Autodesk Inventor part; units mm, degrees
ref_plane "YZ Plane" through (0, 0, 0) normal (1, 0, 0) x (0, 1, 0)
ref_plane "XZ Plane" through (0, 0, 0) normal (0, 1, 0) x (-1, 0, 0)
ref_plane "XY Plane" through (0, 0, 0) normal (0, 0, 1) x (1, 0, 0)
sketch "Эскиз1" plane through (0, 0, 0) normal (0, 1, 0) x (-1, 0, 0)
  line L0 (0, 0) -> (36.1, 0)
  line L1 (36.1, 0) -> (36.1, -7)
  line L2 (36.1, -7) -> (0, -7)
  line L3 (0, -7) -> (0, 0)
  line L4 (36.1, -7) -> (31.1, -7)
  line L5 (31.1, -7) -> (31.1, -12)
  line L6 (31.1, -12) -> (36.1, -12)
  line L7 (36.1, -12) -> (36.1, -7)
  line L8 (36.1, -12) -> (40.1, -12)
  line L9 (40.1, -12) -> (40.1, -5)
  line L10 (40.1, -5) -> (36.1, -5)
  line L11 (36.1, -5) -> (36.1, -12)
  line L12 (18.05, 0) -> (18.05, -7) construction
  line L13 (0, -7) -> (5, -7)
  line L14 (5, -7) -> (5, -12)
  line L15 (5, -12) -> (0, -12)
  line L16 (0, -12) -> (0, -7)
  line L17 (0, -12) -> (-4, -12)
  line L18 (-4, -12) -> (-4, -5)
  line L19 (-4, -5) -> (0, -5)
  line L20 (0, -5) -> (0, -12)
  point P0 (31.1, -7)
  point P1 (0, -5)
  point P2 (36.1, -5)
  dimension "d0" = 36.1
  dimension "d1" = 7
  dimension "d12" = 5
  dimension "d13" = 5
  dimension "d14" = 4
  dimension "d15" = 7
extrude "Выдавливание1" add sketch "Эскиз1" along normal blind 4
sketch "Эскиз2" plane through (0, 0, 0) normal (0, -1, 0) x (1, 0, 0)
  line L0 (-36.1, 0) -> (0, 0) construction
  line L1 (-18.05, 0) -> (-18.05, -7) construction
  line L2 (-5, -7) -> (-31.1, -7) construction
  line L3 (-32.8, -3.5) -> (-3.3, -3.5) construction
  point P0 (-35.5, 0)
  point P1 (0, -7)
  point P2 (-35.5, -7)
  point P3 (-18.05, -3.5)
  dimension "d4" = 29.5
hole "Отверстие1" at (-32.8, 0, -3.5) at (-3.3, 0, -3.5) direction (0, 1, 0) diameter 3.2 end through all countersink diameter 6 countersink angle 90
sketch "Эскиз3" plane through (0, 4, 0) normal (0, 1, 0) x (1, 0, 0)
  line L0 (-40.1, 5) -> (-36.1, 5)
  line L1 (-36.1, 5) -> (-36.1, 12)
  line L2 (-31.1, 12) -> (-40.1, 12)
  line L3 (0, 5) -> (4, 5)
  line L4 (0, 5) -> (0, 12)
  line L5 (4, 12) -> (-5, 12)
  line L6 (4, 5) -> (4, 12)
  line L7 (-40.1, 12) -> (-40.1, 5)
  point P0 (0, 0)
extrude "Выдавливание2" add sketch "Эскиз3" along normal blind 11.05
fillet "Сопряжение1" radius 3.5 4 edges at (-38.1, 15.05, -5) (-38.1, 15.05, -12) (2, 15.05, -5) (2, 15.05, -12)
sketch "Эскиз5" plane through (-40.1, 0, -12) normal (-1, 0, 0) x (0, 0, 1)
  arc A0 (7, 11.55) -> (0, 11.55) centre (3.5, 11.55) ccw
  arc A1 (7, 11.55) -> (0, 11.55) centre (3.5, 11.55) ccw
  point P0 (12, 0)
hole "Отверстие2" at (-40.1, 11.55, -8.5) direction (1, 0, 0) diameter 3.1 depth 3.5
sketch "Эскиз6" plane through (4, 0, -5) normal (1, 0, 0) x (0, 0, -1)
  arc A0 (7, 11.55) -> (0, 11.55) centre (3.5, 11.55) ccw
  point P0 (-5, 0)
hole "Отверстие3" at (4, 11.55, -8.5) direction (-1, 0, 0) diameter 3.1 depth 3.5
sketch "Эскиз7" plane through (-40.1, 0, -12) normal (-1, 0, 0) x (0, 0, 1)
  circle A0 centre (3.5, 11.55) radius 1.55
  line L0 (0.7, 13.1666) -> (3.5, 14.7832)
  line L1 (3.5, 14.7832) -> (6.3, 13.1666)
  line L2 (6.3, 13.1666) -> (6.3, 9.9334)
  line L3 (6.3, 9.9334) -> (3.5, 8.3168)
  line L4 (3.5, 8.3168) -> (0.7, 9.9334)
  line L5 (0.7, 9.9334) -> (0.7, 13.1666)
  line L6 (0, 0) -> (0, 11.55)
  line L7 (0.7, 9.9334) -> (6.3, 9.9334)
  line L8 (6.3, 9.9334) -> (6.3, 0)
  line L9 (6.3, 0) -> (0.7, 0)
  line L10 (0.7, 0) -> (0.7, 9.9334)
  line L11 (0, 0) -> (7, 0)
  point P0 (12, 0)
  point P1 (3.5, 11.55)
  dimension "d33" = 5.6
extrude "Выдавливание3" cut sketch "Эскиз7" along normal blind 3 from surface at -3.5 contours A0 | L0 L1 L2 L7 L5 | L7 L3 L4 | L4 L3 L8 L9 L10
extrude "Выдавливание4" cut sketch "Эскиз7" against normal blind 3 from surface at -40.6 contours A0 | L0 L1 L2 L7 L5 | L7 L3 L4 | L4 L3 L8 L9 L10
sketch "Эскиз8" plane through (0, 4, 0) normal (0, 1, 0) x (1, 0, 0)
  line L0 (-31.1, 7) -> (-31.1, 12)
  line L1 (-31.1, 12) -> (-36.1, 12)
  line L2 (-36.1, 12) -> (-36.1, 10.5)
  line L3 (-36.1, 10.5) -> (-31.1, 10.5)
  line L4 (-31.1, 10.5) -> (-31.1, 12)
  line L5 (-36.1, 12) -> (-36.1, 5)
  point P0 (0, 0)
  dimension "d38" = 1.5
extrude "Выдавливание5" cut sketch "Эскиз8" against normal blind 1.5
properties part number "Крепление OpenMV"
Verification items for the finished model (mm, model axes). A direction names the side the tool comes from. Give positions to 0.01 mm unless a question says otherwise; leave off trailing zeros. Loops run counter-clockwise (first coordinate to the right, second up) from the corner with the lowest first, then second, coordinate; pieces in that order, holes last. Notation, with made-up numbers: M 38,71 L 90,71 A5 cw 90,79 Z; hole C 49.5,-33.75 d11. An arc over 180 degrees is marked long. Return JSON: item names as keys, results as strings.
1) Mould release check, pull along Z, two halves, no side actions. Record for faces 1 (the flat face through (3.5, 6, -9)), 2 (the flat face through (0.5, 7, -9)), 3 (the flat face through (-40.1, 7, -9)), 4 (the flat face through (-18, 2, -7)): released by +Z, released by -Z, zero draft, split by the parting line, or undercut.
Findings:
{"face 1": "undercut", "face 2": "undercut", "face 3": "zero draft", "face 4": "released by -Z"}
2) Section check B-B, the plane x = -32.8. Enter the section's corners in (y, z), and give its area (3 significant figures).
Findings:
{"outline": "M 0,-12 L 2.5,-12 L 2.5,-10.5 L 4,-10.5 L 4,-5.1 L 1.4,-5.1 L 0,-6.5 Z; M 0,-0.5 L 1.4,-1.9 L 4,-1.9 L 4,0 L 0,0 Z", "area": "31.0 mm2"}
3) Section check D-D, the plane x = -3.3. Enter the section's corners in (y, z), and give its area (3 significant figures).
Findings:
{"outline": "M 0,-12 L 4,-12 L 4,-5.1 L 1.4,-5.1 L 0,-6.5 Z; M 0,-0.5 L 1.4,-1.9 L 4,-1.9 L 4,0 L 0,0 Z", "area": "33.2 mm2"}
4) Section check A-A, the plane y = 6.5. Enter the section's corners in (x, z), and give its area (3 significant figures).
Findings:
{"outline": "M -40.1,-12 L -36.1,-12 L -36.1,-5 L -40.1,-5 Z; M 0,-12 L 4,-12 L 4,-5 L 0,-5 Z; hole M -39.6,-11.3 L -36.6,-11.3 L -36.6,-5.7 L -39.6,-5.7 Z; hole M 0.5,-11.3 L 3.5,-11.3 L 3.5,-5.7 L 0.5,-5.7 Z", "area": "22.4 mm2"}
5) Section check C-C, the plane z = -3.5. Enter the section's corners in (x, y).
Findings:
{"outline": "M -36.1,0 L -35.8,0 L -34.4,1.4 L -34.4,4 L -36.1,4 Z; M -31.2,1.4 L -29.8,0 L -6.3,0 L -4.9,1.4 L -4.9,4 L -31.2,4 Z; M -1.7,1.4 L -0.3,0 L 0,0 L 0,4 L -1.7,4 Z"}
6) Tool access check on faces 5 (the flat face through (-34, 3, -10.5)), 6 (the flat face through (-38.079, 13.986, -7.12)), 7 (the cylindrical face through (-39.85, 10.24, -7.67)), 8 (the flat face through (0, 2, -3)). Record the directions out of +Z, -Z, +X, -X, +Y, -Y that give a thin tool (end or side, any length) a straight path to the whole face; none if there is none.
Findings:
{"face 5": "-Z, +Y", "face 6": "-Y", "face 7": "-X", "face 8": "+Z, +X, +Y, -Y"}
7) Gauge pin test, flat ends, axial feed: P1, Ø1.2, axis at x = -12, y = 2.5, coming from the -Z side; P2, Ø3.5, axis at x = -32.8, z = -3.5, coming from the +Y side; P3, Ø1.2, axis at y = 1.5, z = -2.5, coming from the -X side; P4, Ø6, axis at x = -23.5, z = -8.5, coming from the -Y side. Record the tip position at first contact, or that the pin passes through.
Findings:
{"P1": "stops at z = -7", "P2": "stops at y = 4", "P3": "stops at x = -36.1", "P4": "stops at y = 0"}
8) Material ranges on L1, parallel to X at y = 3, z = -3.5; L2, parallel to X at y = 2.75, z = -8.25; L3, parallel to X at y = 10, z = -11.5, recorded low to high. Write a range as [from, to].
Findings:
{"L1": "x = [-36.1, -34.4], [-31.2, -4.9], [-1.7, 0]", "L2": "x = [-40.1, -39.6], [-36.6, -31.1], [-5, 0.5], [3.5, 4]", "L3": "x = [-40.1, -36.1], [0, 4]"}
